The figure shows three views and two pictorial views of one solid part (mm, origin at its lowest corner). Answer the questions. A direction names the side the tool comes from. Give positions to 0.01 mm unless a question says otherwise; leave off trailing zeros. Order: outer loops, then holes, each group sorted by start corner. A loop starts at its lowest first (then second) coordinate and runs counter-clockwise, first axis right, second up. Notation, with made-up numbers: (10.25, 64.5) - (43.25, 64.5) arc R19 cw to (43.25, 69.5) - close; hole circle Ø9 at (77.25, -11). An arc over 180 degrees is marked (long way). Return JSON: item names as keys, results as strings. Group by question number.
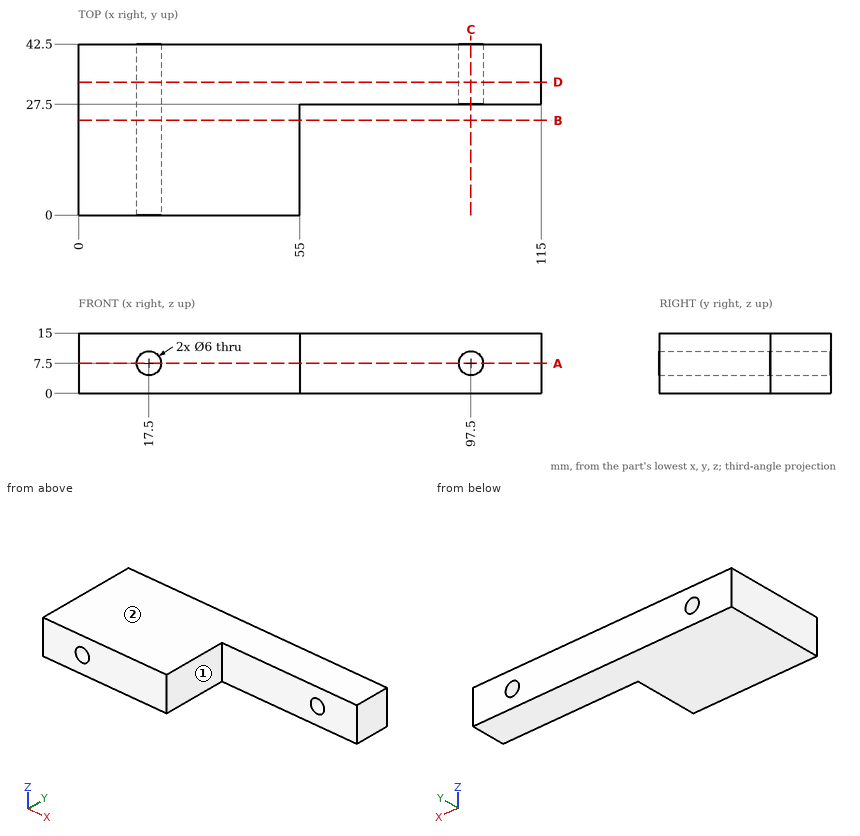
1. The part is cut by section D-D (y = 33). Give the vertices of the cut face in (x, z).
2. Consider probe 1 along X at (y, z) = (35, 7.5); probe 2 along Z at (x, y) = (17.5, 20); probe 3 along X at (y, z) = (19.5, 7.5). Determine where each line is inside the solid, lowest interval first. Write a range as from..to.
3. The part is cut by section C-C (x = 97.5). Give the vertices of the cut face in (y, z).
4. The part is cut by section B-B (y = 23.5). Give the vertices of the cut face in (x, z), and give its area (3 significant figures).
5. A tool of negligible diameter and unlimited length cuts with its end or side. For the marked faces 1 and 2, from which of +Z, -Z, +X, -X, +Y, -Y can it reach the whole face along a straight path? Write none if from no direction.
6. The part is cut by section A-A (z = 7.5). Give the vertices of the cut face in (x, y), and give its area (3 significant figures).
7. Each of these flat-tipped pins is pushed along its axis until it touches: pin 1 (4.5 mm diameter, centred on y = 15.5, z = 8, fed in from +X); pin 2 (4.5 mm diameter, centred on x = 91, z = 4, fed in from -Y). Where does it stop, or does it pass through?
Answers:
{
 "1": {"outline": "(0, 0) - (115, 0) - (115, 15) - (0, 15) - close; hole circle Ø6 at (17.5, 7.5); hole circle Ø6 at (97.5, 7.5)"},
 "2": {"probe 1": "x = 0..14.5, 20.5..94.5, 100.5..115", "probe 2": "z = 0..4.5, 10.5..15", "probe 3": "x = 0..14.5, 20.5..55"},
 "3": {"outline": "(27.5, 0) - (42.5, 0) - (42.5, 4.5) - (27.5, 4.5) - close; (27.5, 10.5) - (42.5, 10.5) - (42.5, 15) - (27.5, 15) - close"},
 "4": {"outline": "(0, 0) - (55, 0) - (55, 15) - (0, 15) - close; hole circle Ø6 at (17.5, 7.5)", "area": "797 mm^2"},
 "5": {"face 1": "+Z, -Z, +X, -Y", "face 2": "+Z, +X, -X, +Y, -Y"},
 "6": {"outline": "(0, 0) - (14.5, 0) - (14.5, 42.5) - (0, 42.5) - close; (20.5, 0) - (55, 0) - (55, 27.5) - (94.5, 27.5) - (94.5, 42.5) - (20.5, 42.5) - close; (100.5, 27.5) - (115, 27.5) - (115, 42.5) - (100.5, 42.5) - close", "area": "2,890 mm^2"},
 "7": {"pin 1": "stops at x = 55", "pin 2": "stops at y = 27.5"}
}
